Drawing for the job (mm, zero at the part's lowest x, y, z). Round coordinates to 2 decimals unless told otherwise and drop trailing zeros. Order: outer loops, then holes, each group sorted by start corner. A loop starts at its lowest first (then second) coordinate and runs counter-clockwise, first axis right, second up. Notation, with made-up numbers: (-11, 82.25) - (43, 82.25) arc R27 ccw to (43, 107.25) - close; hole circle Ø11 at (23, 42.25). An arc over 180 degrees is marked (long way). Put each result on its own line as item: value. Start each with the question number.
Item 1: Mould opens along Z. For the marked faces 1, 2 and 3 say: pulls with the +Z half, pulls with the -Z half, needs draft (parallel to the pull), parting line crosses it, or undercut.
Item 2: Saw through at B-B on x = 36. List the corners of the cut face in (y, z).
Item 3: Saw through at D-D on z = 44.5. List the corners of the cut face in (x, y), plus the area to 3 significant figures.
Item 4: Saw through at A-A on z = 36. List the corners of the cut face in (x, y).
Item 5: Saw through at C-C on y = 12.25. State how many separate pieces and enclosed holes the cut face has, plus the area to 3 significant figures.
Item 6: Pin check, flat tips, straight feed: pin 1 Ø6 at (x, y) = (22.5, 10) entering from +Z (1 decimal); pin 2 Ø1.5 at (y, z) = (17.5, 25.5) entering from -X (1 decimal); pin 3 Ø12 at (y, z) = (18.5, 22.5) entering from -X. Stop position of each tip, or through.
Item 7: Probe probe 1 along X at (y, z) = (6.75, 36); probe 2 along Z at (x, y) = (55, 24) (1 decimal). List the from-to ranges inside material, lowest first.
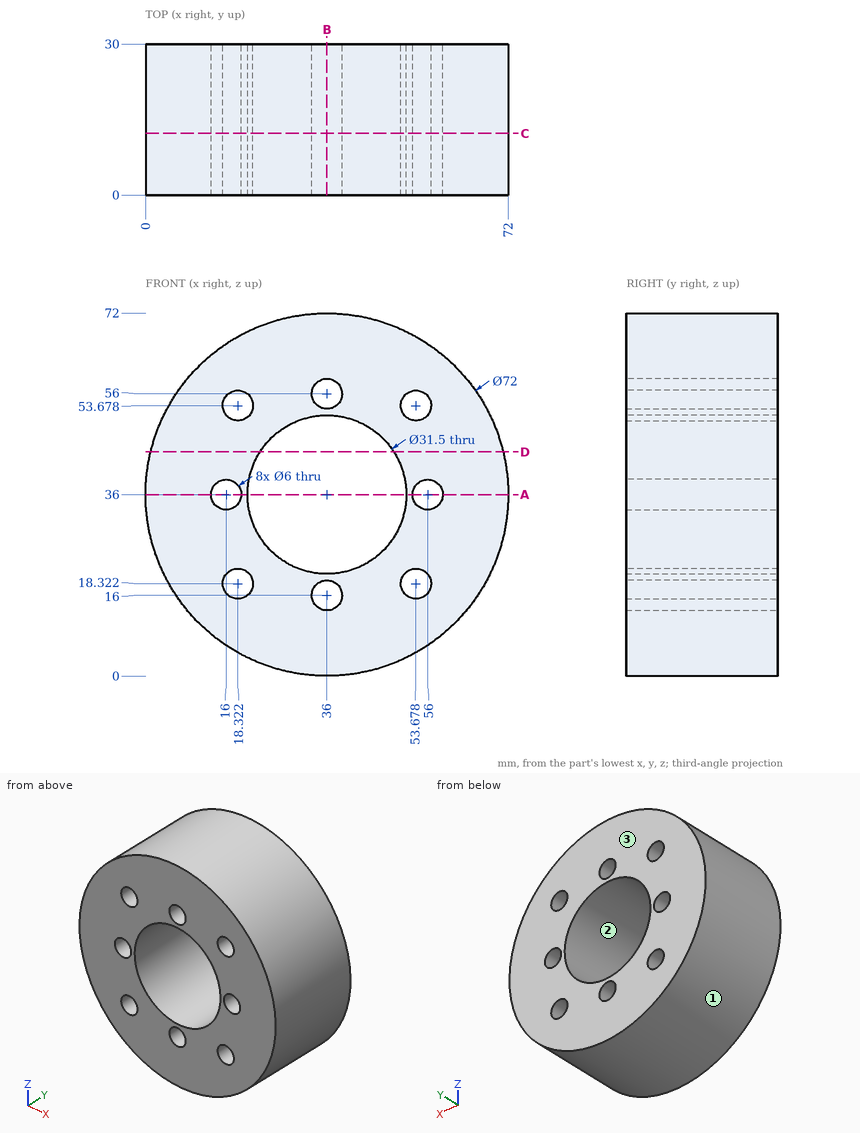
Results found:
1. face 1: parting line crosses it
1. face 2: undercut
1. face 3: needs draft
2. outline: (0, 0) - (30, 0) - (30, 13) - (0, 13) - close; (0, 19) - (30, 19) - (30, 20.25) - (0, 20.25) - close; (0, 51.75) - (30, 51.75) - (30, 53) - (0, 53) - close; (0, 59) - (30, 59) - (30, 72) - (0, 72) - close
3. outline: (1.02, 0) - (22.74, 0) - (22.74, 30) - (1.02, 30) - close; (49.26, 0) - (70.98, 0) - (70.98, 30) - (49.26, 30) - close
3. area: 1,300 mm²
4. outline: (0, 0) - (13, 0) - (13, 30) - (0, 30) - close; (19, 0) - (20.25, 0) - (20.25, 30) - (19, 30) - close; (51.75, 0) - (53, 0) - (53, 30) - (51.75, 30) - close; (59, 0) - (72, 0) - (72, 30) - (59, 30) - close
5. separate pieces: 1
5. enclosed holes: 9
5. area: 3,070 mm²
6. pin 1: stops at z = 70.4
6. pin 2: stops at x = 1.3
6. pin 3: stops at x = 0.79
7. probe 1: x = 0 to 13, 19 to 20.25, 51.75 to 53, 59 to 72
7. probe 2: z = 5.4 to 15.6, 21 to 33.2, 38.8 to 51, 56.4 to 66.6
